```python
from build123d import *

# Parameters (mm, degrees)
BOSS_EXTRUDE1_DEPTH = 60
SKETCH2_W           = 2.3
SKETCH2_H           = 1
CUT_EXTRUDE1_DEPTH  = 10
SKETCH3_W           = 1
SKETCH3_H           = 14
BOSS_EXTRUDE2_DEPTH = 9
SKETCH4_R           = 1.45
CUT_EXTRUDE2_DEPTH  = 9
FILLET1_R           = 0.1
SKETCH5_W           = 7.1
SKETCH5_H           = 5.4
CUT_EXTRUDE3_DEPTH  = 24


with BuildPart() as part:
    # Sketch1 → Boss-Extrude1 (new body)
    with BuildSketch(Plane.XY):
        Polygon((-1.3, 2.75), (-3.6, 2.75), (-3.6, -2.65), (-1.3, -2.65), (-1.3, -1.6), (1.2, -1.6), (1.2, -2.65), (3.5, -2.65), (3.5, 2.75), (1.2, 2.75), (1.2, 1.7), (-1.3, 1.7), align=None)
    extrude(amount=BOSS_EXTRUDE1_DEPTH)

    # Sketch2 → Cut-Extrude1 (cut)
    with BuildSketch(Plane(origin=(0, 2.75, 0), x_dir=(1, 0, 0), z_dir=(0, 1, 0))):
        with Locations((2.35, -3.5)):
            Rectangle(SKETCH2_W, SKETCH2_H)
    extrude(amount=-CUT_EXTRUDE1_DEPTH, mode=Mode.SUBTRACT)

    # Sketch3 → Boss-Extrude2 (add)
    with BuildSketch(Plane(origin=(1.2, 0, 0), x_dir=(0, 0, -1), z_dir=(1, 0, 0))):
        with Locations((-3.5, 0.05)):
            Rectangle(SKETCH3_W, SKETCH3_H)
    extrude(amount=BOSS_EXTRUDE2_DEPTH)

    # Sketch4 → Cut-Extrude2 (cut)
    with BuildSketch(Plane(origin=(0, 0, 3), x_dir=(-1, 0, 0), z_dir=(0, 0, -1))):
        with Locations((-7.5, 0)):
            Circle(SKETCH4_R)
    extrude(amount=-CUT_EXTRUDE2_DEPTH, mode=Mode.SUBTRACT)

    # Fillet1
    fillet1_edges = [part.edges().sort_by_distance(p)[0] for p in [
        (1.2, 2.75, 1.5),
        (1.2, -2.65, 1.5),
        (3.5, 0.05, 3),
        (2.35, -2.65, 3),
        (2.35, 2.75, 3),
        (1.2, -4.8, 3),
        (1.2, 4.9, 3),
        (5.7, -6.95, 3),
        (5.7, 7.05, 3),
        (10.2, 0.05, 3),
        (8.95, 0, 4),
        (8.95, 0, 3),
    ]]
    fillet(fillet1_edges, radius=FILLET1_R)

    # Sketch5 → Cut-Extrude3 (cut)
    with BuildSketch(Plane.XY.offset(60)):
        with Locations((-0.05, 0.05)):
            Rectangle(SKETCH5_W, SKETCH5_H)
    extrude(amount=-CUT_EXTRUDE3_DEPTH, mode=Mode.SUBTRACT)


solid = part.part
```
Model file for the job. Use its own axes, mm. A direction names the side the tool comes from. Round coordinates to 2 decimals unless told otherwise and drop trailing zeros. Order: outer loops, then holes, each group sorted by start corner. A loop starts at its lowest first (then second) coordinate and runs counter-clockwise, first axis right, second up. Notation, with made-up numbers: M 9,13.25 L 25,13.25 A12 cw 25,20.25 Z; hole C 51.5,-28 d2. An arc over 180 degrees is marked long. Use CSV: the item, a comma, the result in double quotes.
Item 1: Pin check, flat tips, straight feed: pin 1 (1 mm diameter, centred on x = -2, z = 14.5, fed in from -Y); pin 2 (2 mm diameter, centred on x = 0, z = 22, fed in from -Y); pin 3 (1.6 mm diameter, centred on y = 4.5, z = 26.5, fed in from -X); pin 4 (2.5 mm diameter, centred on x = 6.5, y = -3.5, fed in from +Z). Stop position of each tip, or through.
Worked answers:
pin 1,"y = -2.65"
pin 2,"y = -1.6"
pin 3,"through"
pin 4,"z = 4"
Item 2: Which spindle directions (+Z, -Z, +X, -X, +Y, -Y) get a long thin tool onto all of the face, cutting with end or side? Do faces 1 (the face through (1.2, -2, 17)), 2 (the face through (-1.3, 2, 18)), 3 (the face through (2, 2.75, 20)), 4 (the face through (2, -2.65, 20)). Say none if no direction does.
Worked answers:
face 1,"+Z, -Z, -Y"
face 2,"+Z, -Z, +Y"
face 3,"+Z, +X, -X, +Y"
face 4,"+Z, +X, -X, -Y"
Item 3: Saw through at B-B (x = 7.5). List the corners of the cut face in (y, z).
Worked answers:
outline,"M -6.95,3.1 A0.1 ccw -6.85,3 L -1.55,3 A0.1 ccw -1.45,3.1 L -1.45,3.9 A0.1 ccw -1.55,4 L -6.95,4 Z; M 1.45,3.1 A0.1 ccw 1.55,3 L 6.95,3 A0.1 ccw 7.05,3.1 L 7.05,4 L 1.55,4 A0.1 ccw 1.45,3.9 Z"
Item 4: Saw through at C-C (z = 31). List the corners of the cut face in (x, y), plus the area to 3 significant figures.
Worked answers:
outline,"M -3.6,-2.65 L -1.3,-2.65 L -1.3,-1.6 L 1.2,-1.6 L 1.2,-2.65 L 3.5,-2.65 L 3.5,2.75 L 1.2,2.75 L 1.2,1.7 L -1.3,1.7 L -1.3,2.75 L -3.6,2.75 Z"
area,"33.1 mm²"
Item 5: Saw through at A-A (y = 0). List the corners of the cut face in (x, z).
Worked answers:
outline,"M -3.6,0 L 3.5,0 L 3.5,2.9 A0.1 cw 3.6,3 L 5.95,3 A0.1 ccw 6.05,3.1 L 6.05,3.9 A0.1 ccw 5.95,4 L 3.5,4 L 3.5,36 L -3.6,36 Z; M 8.95,3.1 A0.1 ccw 9.05,3 L 10.1,3 A0.1 ccw 10.2,3.1 L 10.2,4 L 9.05,4 A0.1 ccw 8.95,3.9 Z"
Item 6: Probe probe 1 along Y at (x, z) = (7.5, 3.45); probe 2 along Z at (x, y) = (6.25, 6.25); probe 3 along Y at (x, z) = (-1, 20). List the from-to ranges inside material, lowest first.
Worked answers:
probe 1,"-6.95 to -1.45, 1.45 to 7.05"
probe 2,"3 to 4"
probe 3,"-1.6 to 1.7"
Item 7: Saw through at D-D (y = 3.25). List the corners of the cut face in (x, z).
Worked answers:
outline,"M 1.2,3.1 A0.1 ccw 1.3,3 L 10.1,3 A0.1 ccw 10.2,3.1 L 10.2,4 L 1.2,4 Z"
Item 8: Pull direction X, two halves, no side cores. Call faces 5 (the face through (-3.6, 0, 18)), 6 (the face through (0, -1.6, 18)), 7 (the face through (2, 2.75, 1)): released by +X, released by -X, zero draft, split by the parting line, or undercut.
Worked answers:
face 5,"released by -X"
face 6,"undercut"
face 7,"zero draft"
